from build123d import *

# Parameters (mm, degrees)
TAGLIO_ESTRUSIONE1_REACH             = 10
SCHIZZO2_W                           = 1.5
SCHIZZO2_H                           = 8
TAGLIO_ESTRUSIONE1_DIRECTION_2_REACH = 10
SCHIZZO7_R                           = 3
TAGLIO_ESTRUSIONE2_DEPTH             = 41
FORO_FILETTATO_M8_1_D                = 6.8
FORO_FILETTATO_M8_1_DEPTH            = 12
FORO_FILETTATO_M8_1_TIP              = 2.042926105
SCHIZZO10_OUTSIDE_W                  = 27.192
SCHIZZO10_OUTSIDE_H                  = 27.192
SCHIZZO10_OUTSIDE_R                  = 6
TAGLIO_ESTRUSIONE3_DEPTH             = 13


with BuildPart() as part:
    # Schizzo1 → Rivoluzione1 (revolve)
    with BuildSketch(Plane.XY):
        Polygon((0, 0), (-5, 0), (-8, 1.5), (-8, 12), (-6, 12), (-6, 13.5), (-8, 13.5), (-8, 15), (-6, 15), (-6, 16.5), (-8, 16.5), (-8, 18), (-6, 18), (-6, 19.5), (-8, 19.5), (-8, 27), (-8, 40), (0, 40), align=None)
    revolve(axis=Axis((0, 129.407380346, 0), (0, -1, 0)))

    # Schizzo2 → Taglio-Estrusione1 (cut, up to next)
    with BuildSketch(Plane.XY, mode=Mode.PRIVATE) as taglio_estrusione1_sk1:
        with Locations((-7.25, 4)):
            Rectangle(SCHIZZO2_W, SCHIZZO2_H)
    taglio_estrusione1_tool1 = extrude(taglio_estrusione1_sk1.sketch, amount=-TAGLIO_ESTRUSIONE1_REACH, mode=Mode.PRIVATE) & part.part
    add(taglio_estrusione1_tool1.solids().sort_by_distance((-7.25, 4, 0))[0], mode=Mode.SUBTRACT)
    # Schizzo2 → Taglio-Estrusione1 (cut, up to next)
    with BuildSketch(Plane.XY, mode=Mode.PRIVATE) as taglio_estrusione1_sk2:
        with Locations((7.25, 4)):
            Rectangle(SCHIZZO2_W, SCHIZZO2_H)
    taglio_estrusione1_tool2 = extrude(taglio_estrusione1_sk2.sketch, amount=-TAGLIO_ESTRUSIONE1_REACH, mode=Mode.PRIVATE) & part.part
    add(taglio_estrusione1_tool2.solids().sort_by_distance((7.25, 4, 0))[0], mode=Mode.SUBTRACT)

    # Schizzo2 → Taglio-Estrusione1 direction 2 (cut, up to next)
    with BuildSketch(Plane.XY, mode=Mode.PRIVATE) as taglio_estrusione1_direction_2_sk1:
        with Locations((-7.25, 4)):
            Rectangle(SCHIZZO2_W, SCHIZZO2_H)
    taglio_estrusione1_direction_2_tool1 = extrude(taglio_estrusione1_direction_2_sk1.sketch, amount=TAGLIO_ESTRUSIONE1_DIRECTION_2_REACH, mode=Mode.PRIVATE) & part.part
    add(taglio_estrusione1_direction_2_tool1.solids().sort_by_distance((-7.25, 4, 0))[0], mode=Mode.SUBTRACT)
    # Schizzo2 → Taglio-Estrusione1 direction 2 (cut, up to next)
    with BuildSketch(Plane.XY, mode=Mode.PRIVATE) as taglio_estrusione1_direction_2_sk2:
        with Locations((7.25, 4)):
            Rectangle(SCHIZZO2_W, SCHIZZO2_H)
    taglio_estrusione1_direction_2_tool2 = extrude(taglio_estrusione1_direction_2_sk2.sketch, amount=TAGLIO_ESTRUSIONE1_DIRECTION_2_REACH, mode=Mode.PRIVATE) & part.part
    add(taglio_estrusione1_direction_2_tool2.solids().sort_by_distance((7.25, 4, 0))[0], mode=Mode.SUBTRACT)

    # Schizzo7 → Taglio-Estrusione2 (cut, through all)
    with BuildSketch(Plane(origin=(0, 40, 0), x_dir=(1, 0, 0), z_dir=(0, 1, 0))):
        Circle(SCHIZZO7_R)
    extrude(amount=-TAGLIO_ESTRUSIONE2_DEPTH, mode=Mode.SUBTRACT)

    # Foro filettato M8-1
    with Locations(Plane(origin=(0, 0, 0), x_dir=(-1, 0, 0), z_dir=(0, -1, 0))):
        with Locations((0, 0)):
            Hole(FORO_FILETTATO_M8_1_D / 2, depth=FORO_FILETTATO_M8_1_DEPTH)
            with Locations((0, 0, -(FORO_FILETTATO_M8_1_DEPTH + FORO_FILETTATO_M8_1_TIP / 2))):  # 118° drill point
                Cone(0, FORO_FILETTATO_M8_1_D / 2, FORO_FILETTATO_M8_1_TIP, mode=Mode.SUBTRACT)

    # Schizzo10 outside → Taglio-Estrusione3 (cut)
    with BuildSketch(Plane(origin=(0, 40, 0), x_dir=(1, 0, 0), z_dir=(0, 1, 0))):
        Rectangle(SCHIZZO10_OUTSIDE_W, SCHIZZO10_OUTSIDE_H)
        Circle(SCHIZZO10_OUTSIDE_R, mode=Mode.SUBTRACT)
    extrude(amount=-TAGLIO_ESTRUSIONE3_DEPTH, mode=Mode.SUBTRACT)


solid = part.part
Build history of the part. All positions in model axes, mm. A direction names the side the tool comes from. Round coordinates to 2 decimals unless told otherwise and drop trailing zeros. Write each loop counter-clockwise with the first axis right and the second up, starting at its lowest first coordinate (ties: lowest second). Pieces come first, ordered by that corner, then holes. Notation, with made-up numbers: (85, -13) - (92, -13) arc R29 cw to (92, 15) - close; hole circle Ø8 at (14.5, 26.25). An arc over 180 degrees is marked (long way). One line per question, with ' | ' between items.
1. Drill centre lines: line 1 along Z through (x, y) = (0, 29.5); line 2 along Y through (x, z) = (5.75, 4.75); line 3 along Y through (x, z) = (-4.25, 4.5). Where is each one in solid material? Low to high. Write a range as from..to.
Results are:
line 1: -6..-3, 3..6 | line 2: 1.23..12, 13.5..15, 16.5..18, 19.5..27 | line 3: 0.59..12, 13.5..15, 16.5..18, 19.5..27
2. Mould opens along X. For faces 1 (the face through (2, 18, -6)), 2 (the face through (1.73, 17.26, 7.81)), 3 (the face through (-0.74, 6.08, 3.32)) say: released by +X, released by -X, zero draft, split by the parting line, or undercut.
Results are:
face 1: zero draft | face 2: split by the parting line | face 3: undercut
3. Band-saw the part on B-B, the plane z = -6.75. Give the number of separate pieces and of enclosed holes in the cut face, and give its area (3 significant figures).
Results are:
separate pieces: 4 | enclosed holes: 0 | area: 184 mm^2
4. Drop flat-ended pins along their axis: pin 1 Ø8 at (y, z) = (3.5, -0.5) entering from -X; pin 2 Ø1.2 at (x, z) = (7.5, 0) entering from -Y; pin 3 Ø5 at (y, z) = (10.5, -5) entering from -X. Give the stop position or say it passes through.
Results are:
pin 1: x = -6.5 | pin 2: y = 8 | pin 3: x = -7.6
5. Tool access for faces 4 (the face through (7, 8, 0)), 5 (the face through (-7, 8, 0)), 6 (the face through (6, 19, 0)): list every direction of +Z, -Z, +X, -X, +Y, -Y with a clear straight run to the whole face (end or side of a thin tool).
Results are:
face 4: +Z, -Z, +X, -Y | face 5: +Z, -Z, -X, -Y | face 6: none
6. Band-saw the part on C-C, the plane y = 28.5. Write the cut outline in (x, z), and give its area (3 significant figures).
Results are:
outline: circle Ø12 at (0, 0); hole circle Ø6 at (0, 0) | area: 84.8 mm^2
7. Band-saw the part on A-A, the plane y = 3. Write the cut outline in (x, z), and give its area (3 significant figures).
Results are:
outline: (-6.5, -4.66) arc R8 ccw to (6.5, -4.66) - (6.5, 4.66) arc R8 ccw to (-6.5, 4.66) - close; hole circle Ø6.8 at (0, 0) | area: 146 mm^2
